Verification items for this drawing (mm, ordinates from the low corner). A direction names the side the tool comes from. Give positions to 0.01 mm unless a question says otherwise; leave off trailing zeros. Loops run counter-clockwise (first coordinate to the right, second up) from the corner with the lowest first, then second, coordinate; pieces in that order, holes last. Notation, with made-up numbers: M 2,-30 L 49,-30 A22 cw 49,5 Z; hole C -29,-7 d4. An arc over 180 degrees is marked long. Use a Markdown table: item, result.
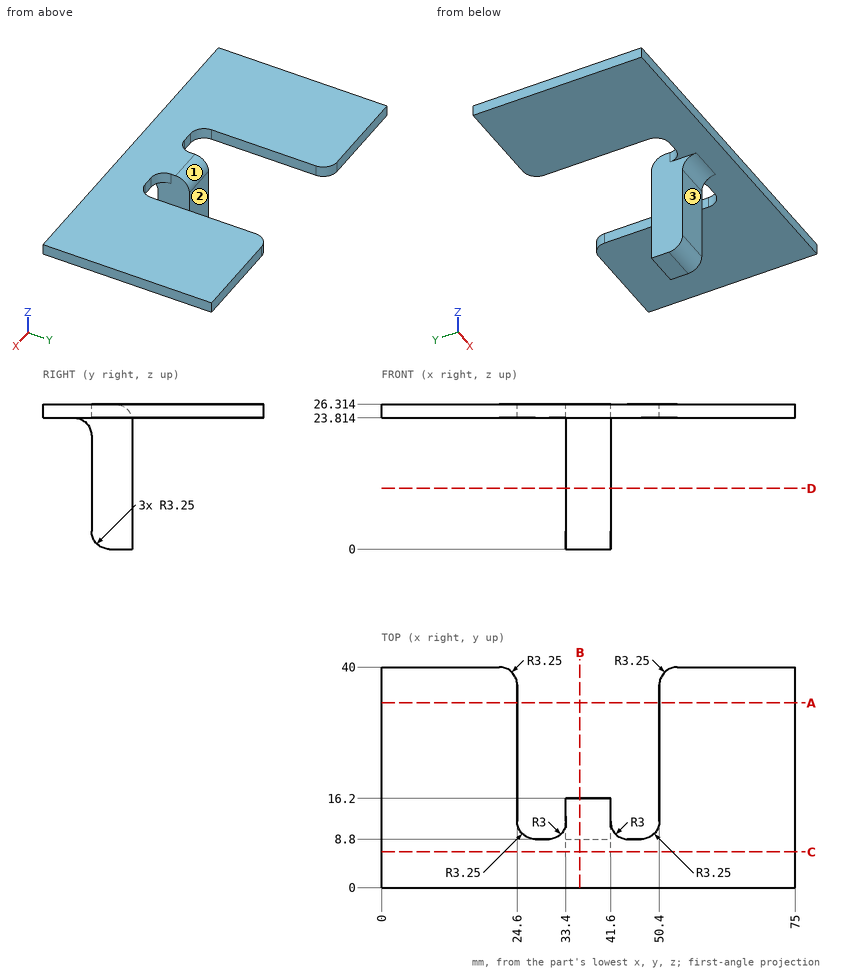
(1) Set-up check for the marked faces 1, 2 and 3: record each of +Z, -Z, +X, -X, +Y, -Y from which the full face is reachable in a straight line by a thin tool's end or side.
Results below:
| item | result |
|---|---|
| face 1 | +Z, +Y |
| face 2 | +Z, -Z, +X, -X, +Y |
| face 3 | -Z, +X, -X, -Y |
(2) Cross-section at D-D on z = 11. Record the cut outline in (x, y).
Results below:
| item | result |
|---|---|
| outline | M 33.4,8.8 L 41.6,8.8 L 41.6,16.2 L 33.4,16.2 Z |
(3) Cross-section at C-C on y = 6.5. Record the cut outline in (x, z), then the cut area to 3 significant figures.
Results below:
| item | result |
|---|---|
| outline | M 0,23.81 L 33.4,23.81 L 33.4,23.67 L 41.6,23.67 L 41.6,23.81 L 75,23.81 L 75,26.31 L 0,26.31 Z |
| area | 189 mm^2 |
(4) Cross-section at A-A on y = 33.5. Record the cut outline in (x, z), then the cut area to 3 significant figures.
Results below:
| item | result |
|---|---|
| outline | M 0,23.81 L 24.6,23.81 L 24.6,26.31 L 0,26.31 Z; M 50.4,23.81 L 75,23.81 L 75,26.31 L 50.4,26.31 Z |
| area | 123 mm^2 |
(5) Gauge pin test, flat ends, axial feed: P1, Ø3, axis at y = 12, z = 8, coming from the +X side; P2, Ø3, axis at y = 8, z = 19.5, coming from the -X side; P3, Ø4, axis at x = 35.5, z = 6.5, coming from the +Y side. Record the tip position at first contact, or that the pin passes through.
Results below:
| item | result |
|---|---|
| P1 | x = 41.6 |
| P2 | x = 33.4 |
| P3 | y = 16.2 |
(6) Material ranges on line 1 (Z direction, x = 26.5, y = 7.5); line 2 (X direction, y = 9.5, z = 9), recorded low to high.
Results below:
| item | result |
|---|---|
| line 1 | 23.81 to 26.31 |
| line 2 | 33.4 to 41.6 |
(7) Cross-section at B-B on x = 36. Record the cut outline in (y, z), then the cut area to 3 significant figures.
Results below:
| item | result |
|---|---|
| outline | M 0,23.81 L 5.55,23.81 A3.25 cw 8.8,20.56 L 8.8,3.25 A3.25 ccw 12.05,0 L 16.2,0 L 16.2,23.06 A3.25 ccw 12.95,26.31 L 0,26.31 Z |
| area | 214 mm^2 |
